Geometry check sheet. Reference: the model listing, model coordinates, mm. Face numbers are marked on the shaded views. A direction names the side the tool comes from. Round coordinates to 2 decimals unless told otherwise and drop trailing zeros. Write each loop counter-clockwise with the first axis right and the second up, starting at its lowest first coordinate (ties: lowest second). Pieces come first, ordered by that corner, then holes. Notation, with made-up numbers: (62.25, 47) -> (94.25, 47) arc R28 ccw to (94.25, 85) -> close; hole circle Ø3 at (34, 87.5). An arc over 180 degrees is marked (long way). Use a Markdown table: item, result.
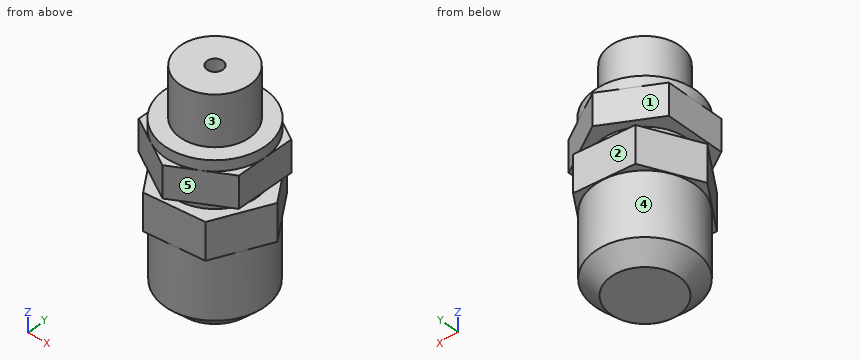
```python
from build123d import *

# Parameters (mm, degrees)
BASE_EXTRUDE_DEPTH  = 6
SKETCH2_R           = 9.5
BOSS_EXTRUDE1_DEPTH = 2
SKETCH3_R           = 6.5785
BOSS_EXTRUDE2_DEPTH = 9.5
SKETCH4_R           = 1.5
CUT_EXTRUDE1_DEPTH  = 9.5
SKETCH5_R           = 8
BOSS_EXTRUDE3_DEPTH = 2
BOSS_EXTRUDE4_DEPTH = 7
SKETCH8_R           = 9.4
BOSS_EXTRUDE5_DEPTH = 15
CHAMFER1_SIZE       = 3


with BuildPart() as part:
    # Sketch1 → Base-Extrude (new body)
    with BuildSketch(Plane.XY):
        Polygon((0, 10.969655115), (-9.5, 5.484827557), (-9.5, -5.484827557), (0, -10.969655115), (9.5, -5.484827557), (9.5, 5.484827557), align=None)
    extrude(amount=BASE_EXTRUDE_DEPTH)

    # Sketch2 → Boss-Extrude1 (add)
    with BuildSketch(Plane.XY.offset(6)):
        Circle(SKETCH2_R)
    extrude(amount=BOSS_EXTRUDE1_DEPTH)

    # Sketch3 → Boss-Extrude2 (add)
    with BuildSketch(Plane.XY.offset(8)):
        Circle(SKETCH3_R)
    extrude(amount=BOSS_EXTRUDE2_DEPTH)

    # Sketch4 → Cut-Extrude1 (cut)
    with BuildSketch(Plane.XY.offset(17.5)):
        Circle(SKETCH4_R)
    extrude(amount=-CUT_EXTRUDE1_DEPTH, mode=Mode.SUBTRACT)

    # Sketch5 → Boss-Extrude3 (add)
    with BuildSketch(Plane(origin=(0, 0, 0), x_dir=(-1, 0, 0), z_dir=(0, 0, -1))):
        Circle(SKETCH5_R)
    extrude(amount=BOSS_EXTRUDE3_DEPTH)

    # Sketch7 → Boss-Extrude4 (add)
    with BuildSketch(Plane(origin=(0, 0, -2), x_dir=(-1, 0, 0), z_dir=(0, 0, -1))):
        Polygon((10.924605006, -0.99314591), (6.32239209, 8.964412507), (-4.602212916, 9.957558416), (-10.924605006, 0.99314591), (-6.32239209, -8.964412507), (4.602212916, -9.957558416), align=None)
    extrude(amount=BOSS_EXTRUDE4_DEPTH)

    # Sketch8 → Boss-Extrude5 (add)
    with BuildSketch(Plane(origin=(0, 0, -9), x_dir=(-1, 0, 0), z_dir=(0, 0, -1))):
        Circle(SKETCH8_R)
    extrude(amount=BOSS_EXTRUDE5_DEPTH)

    # Chamfer1
    chamfer1_edges = [part.edges().sort_by_distance(p)[0] for p in [
        (9.4, 0, -24),
    ]]
    chamfer(chamfer1_edges, length=CHAMFER1_SIZE)


solid = part.part
```
(1) Gauge pin test, flat ends, axial feed: pin 1 Ø4 at (x, z) = (2, -12.5) entering from +Y; pin 2 Ø6 at (x, z) = (-3, 6.5) entering from +Y; pin 3 Ø8 at (y, z) = (-5.5, 2.5) entering from -X; pin 4 Ø4 at (x, y) = (-6, -3.5) entering from +Z. Record the tip position at first contact, or that the pin passes through.
A:
| item | result |
|---|---|
| pin 1 | stops at y = 9.4 |
| pin 2 | stops at y = 10.95 |
| pin 3 | stops at x = -9.5 |
| pin 4 | stops at z = 17.5 |
(2) Section check A-A on z = 4.5. Record the cut outline in (x, y).
A:
| item | result |
|---|---|
| outline | (-9.5, -5.48) -> (0, -10.97) -> (9.5, -5.48) -> (9.5, 5.48) -> (0, 10.97) -> (-9.5, 5.48) -> close |
(3) Thickness scan on line 1 (Y direction, x = 0, z = 10.75); line 2 (X direction, y = 1.25, z = 13); line 3 (Z direction, x = -9, y = 5). Record the ranges inside material, lowest first.
A:
| item | result |
|---|---|
| line 1 | y = -6.58 to -1.5, 1.5 to 6.58 |
| line 2 | x = -6.46 to -0.83, 0.83 to 6.46 |
| line 3 | z = 0 to 6 |
(4) Access from +Z, -Z, +X, -X, +Y, -Y to the whole of each face (thin tool, end or side, straight path). Record for the marked faces 1, 2, 3, 4 and 5.
A:
| item | result |
|---|---|
| face 1 | +Z, -X, +Y |
| face 2 | -Z, -X, +Y |
| face 3 | +Z |
| face 4 | -Z |
| face 5 | +Z, +X, -Y |
(5) Section check B-B on z = 10. Record the cut outline in (x, y), plus the area to 3 significant figures.
A:
| item | result |
|---|---|
| outline | circle Ø13.16 at (0, 0); hole circle Ø3 at (0, 0) |
| area | 129 mm2 |
